Print and shaded views of the part. All mm, measured from the part's lowest x, y and z. A direction names the side the tool comes from. Coordinates: 2 decimals unless noted, no trailing zeros. Loops run counter-clockwise (first coordinate to the right, second up) from the corner with the lowest first, then second, coordinate; pieces in that order, holes last. Notation, with made-up numbers: (36, 23) -> (50, 23) arc R4 cw to (50, 29) -> close; hole circle Ø3 at (57, 40). An arc over 180 degrees is marked (long way). One line per item, written item: value. Start each with the question number.
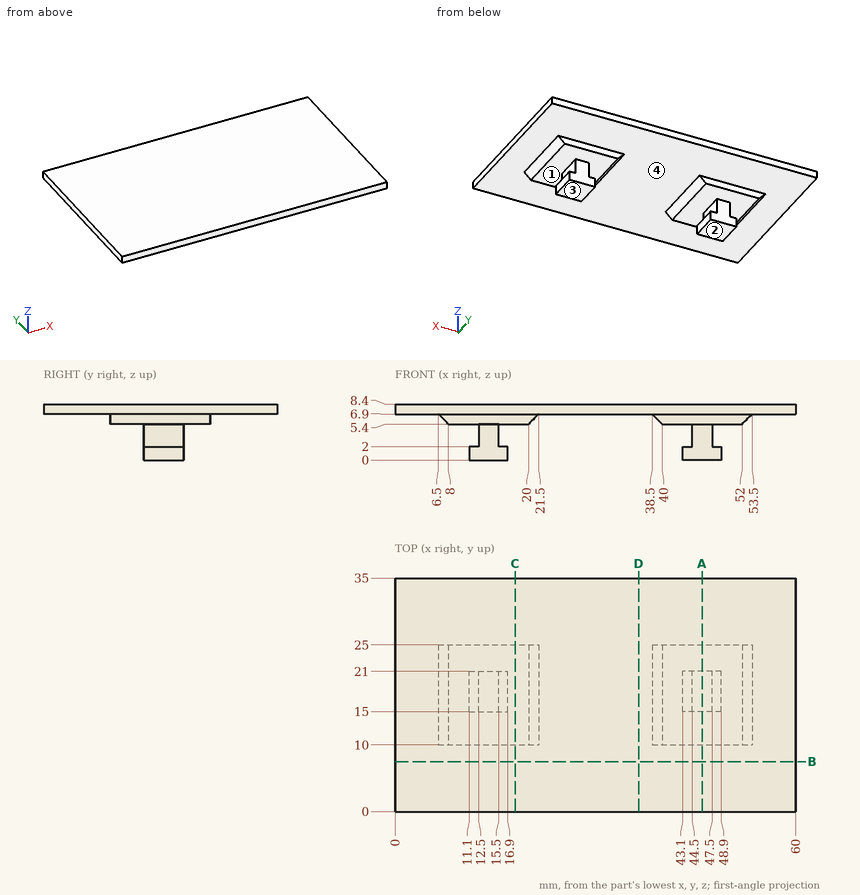
1) Probe line 1 (X direction, y = 20, z = 1.5); line 2 (Z direction, x = 37, y = 17); line 3 (Z direction, x = 47.5, y = 14.5). List the from-to ranges inside material, lowest first. Write a range as from..to.
2) Pull direction X, two halves, no side cores. Call the marked faces 1 and 2: +X half, -X half, draft (parallel to the pull), parting line (faces both ways), or undercut.
3) Slice it at D-D (x = 36.5). Give the cut face in (y, z).
4) Pin check, flat tips, straight feed: pin 1 Ø1.7 at (x, z) = (11.5, 6) entering from -Y; pin 2 Ø1 at (y, z) = (18, 1.5) entering from -X; pin 3 Ø4 at (x, z) = (42, 2) entering from -Y. Stop position of each tip, or through.
5) Tool access for the marked faces 3 and 4: list every direction of +Z, -Z, +X, -X, +Y, -Y with a clear straight run to the whole face (end or side of a thin tool).
6) Slice it at C-C (x = 18). Give the cut face in (y, z), then the cut area to 3 significant figures.
7) Slice it at B-B (y = 7.5). Give the cut face in (x, z), then the cut area to 3 significant figures.
8) Slice it at A-A (x = 46). Give the cut face in (y, z), then the cut area to 3 significant figures.
Check sheet entries:
1. line 1: x = 11.1..16.9, 43.1..48.9
1. line 2: z = 6.9..8.4
1. line 3: z = 5.4..8.4
2. face 1: undercut
2. face 2: draft
3. outline: (0, 6.9) -> (35, 6.9) -> (35, 8.4) -> (0, 8.4) -> close
4. pin 1: stops at y = 10
4. pin 2: stops at x = 11.1
4. pin 3: stops at y = 15
5. face 3: -Z, +X, -X, +Y, -Y
5. face 4: -Z
6. outline: (0, 6.9) -> (10, 6.9) -> (10, 5.4) -> (25, 5.4) -> (25, 6.9) -> (35, 6.9) -> (35, 8.4) -> (0, 8.4) -> close
6. area: 75.0 mm^2
7. outline: (0, 6.9) -> (60, 6.9) -> (60, 8.4) -> (0, 8.4) -> close
7. area: 90.0 mm^2
8. outline: (0, 6.9) -> (10, 6.9) -> (10, 5.4) -> (15, 5.4) -> (15, 0) -> (21, 0) -> (21, 5.4) -> (25, 5.4) -> (25, 6.9) -> (35, 6.9) -> (35, 8.4) -> (0, 8.4) -> close
8. area: 107 mm^2
